from build123d import *

# Parameters (mm, degrees)
BASE_FLANGE1_DEPTH = 63.5


# Sheet-metal steps are written as plain solids
with BuildPart() as part:
    # Sketch1 → Base-Flange1 (new, symmetric)
    with BuildSketch(Plane.XY):
        with BuildLine():
            ThreePointArc((265, 308.636973764), (248.140563862, 281.667999342), (216.511627907, 285.011138385))
            ThreePointArc((216.511627907, 285.011138385), (-205.207518157, 329.586325632), (-430, -30))
            ThreePointArc((-430, -30), (-295.269119346, -355.269119346), (30, -490))
            ThreePointArc((30, -490), (397.695526217, -337.695526217), (550, 30))
            Line((550, 30), (550, 308.636973764))
            Line((550, 308.636973764), (546, 308.636973764))
            Line((546, 308.636973764), (546, 30))
            ThreePointArc((546, 30), (394.867099092, -334.867099092), (30, -486))
            ThreePointArc((30, -486), (-292.440692221, -352.440692221), (-426, -30))
            ThreePointArc((-426, -30), (-203.455442975, 325.990462376), (214.046511628, 281.861027001))
            ThreePointArc((214.046511628, 281.861027001), (249.892639043, 278.072136085), (269, 308.636973764))
            Line((269, 308.636973764), (265, 308.636973764))
        make_face()
    extrude(amount=BASE_FLANGE1_DEPTH, both=True)


solid = part.part
The model under review builds one solid part; all positions refer to its coordinate system, in mm. A direction names the side the tool comes from. Give positions to 0.01 mm unless a question says otherwise; leave off trailing zeros. Order: outer loops, then holes, each group sorted by start corner. A loop starts at its lowest first (then second) coordinate and runs counter-clockwise, first axis right, second up. Notation, with made-up numbers: (48, -39.5) -> (78, -39.5) arc R32 cw to (78, -1.5) -> close; hole circle Ø8 at (12, 32.25). An arc over 180 degrees is marked (long way). Write item = value, one per line. Start each with the question number.
(1) Tool access review of faces 1 (the flat face through (546, 171, 1)), 2 (the cylindrical face through (-288.876, -355.967, 0.889)), 3 (the flat face through (550, 167, 1)): name each direction out of +Z, -Z, +X, -X, +Y, -Y from which nothing blocks a thin tool from reaching the whole face with its end or side.
(2) Take a section at D-D (x = 313.5). Write out the cut boundary in (y, z), plus the area to 3 significant figures.
(3) Draft analysis for pull direction X (two halves, no side actions). For faces 4 (the cylindrical face through (249.41, 277.84, 0.89)), 5 (the cylindrical face through (-298.8, -351.7, 0.9)), 6 (the cylindrical face through (393.63, -341.716, 0.889)), state which applies: +X half, -X half, draft (parallel to the pull), parting line (faces both ways), or undercut.
(4) For L1, parallel to X at y = 292, z = -41; L2, parallel to X at y = 296, z = -2.5; L3, parallel to X at y = -246, z = 42.5, list the stretches that pass through material, from the lowest coordinate up. Write a range as from..to.
(5) Take a section at A-A (y = -378). Write out the cut boundary in (x, z).
(6) Take a section at B-B (x = -344). Write out the cut boundary in (y, z).
(7) For pin 1 Ø3 at (y, z) = (104, -17) entering from -X; pin 2 Ø1.2 at (x, z) = (548, 17.5) entering from +Y; pin 3 Ø6 at (y, z) = (-100.5, -48.5) entering from +X, all flat-tipped, find the tip position at first contact; note any pin that passes through.
(8) Take a section at C-C (z = -36). Write out the cut boundary in (x, y).
Returned:
q1.face_1 = +Z, -Z, +Y
q1.face_2 = +Z, -Z
q1.face_3 = +Z, -Z, +X, +Y, -Y
q2.outline = (-405.92, -63.5) -> (-401.14, -63.5) -> (-401.14, 63.5) -> (-405.92, 63.5) -> close
q2.area = 607 mm²
q3.face_4 = undercut
q3.face_5 = -X half
q3.face_6 = +X half
q4.L1 = -267.31..-260.5, 200.5..207.31, 259.96..264.65, 546..550
q4.L2 = -261.78..-254.81, 194.81..201.78, 262.21..266.56, 546..550
q4.L3 = -376.13..-371.6, 465.98..470.71
q5.outline = (-270.83, -63.5) -> (-264.67, -63.5) -> (-264.67, 63.5) -> (-270.83, 63.5) -> close; (345.9, -63.5) -> (352.39, -63.5) -> (352.39, 63.5) -> (345.9, 63.5) -> close
q6.outline = (-297.81, -63.5) -> (-290.88, -63.5) -> (-290.88, 63.5) -> (-297.81, 63.5) -> close; (211.29, -63.5) -> (217.8, -63.5) -> (217.8, 63.5) -> (211.29, 63.5) -> close
q7.pin_1 = -407.42
q7.pin_2 = 308.64
q7.pin_3 = 534.13
q8.outline = (-430, -30) arc R460 ccw to (30, -490) arc R520 ccw to (550, 30) -> (550, 308.64) -> (546, 308.64) -> (546, 30) arc R516 cw to (30, -486) arc R456 cw to (-426, -30) arc R396 cw to (214.05, 281.86) arc R34 ccw to (269, 308.64) -> (265, 308.64) arc R30 cw to (216.51, 285.01) arc R400 ccw to start
